Geometry: final body of the model. Coordinates: model frame, mm. A direction names the side the tool comes from. Give positions to 0.01 mm unless a question says otherwise; leave off trailing zeros. Loops run counter-clockwise (first coordinate to the right, second up) from the corner with the lowest first, then second, coordinate; pieces in that order, holes last. Notation, with made-up numbers: (19.25, 26) - (42.25, 26) arc R33 ccw to (42.25, 56) - close; hole circle Ø8 at (-2, -22.75). An arc over 180 degrees is marked (long way). Answer in a Markdown table with one row per item.
from build123d import *

# Parameters (mm, degrees)
F0_R     = 3.81
F1_DEPTH = 5.588
F2_DEPTH = 3.81
F3_R     = 1.5875
F4_DEPTH = 76.2
F5_SIZE  = 0.254
F6_SIZE  = 0.254


with BuildPart() as f1:
    # F0 (on Front) → F1 (new body)
    with BuildSketch(Plane.XZ):
        Circle(F0_R)
        Polygon((0, 2.54), (2.199705, 1.27), (2.199705, -1.27), (0, -2.54), (-2.199705, -1.27), (-2.199705, 1.27), align=None, mode=Mode.SUBTRACT)
    extrude(amount=F1_DEPTH)

    # F0 (on Front) → F2 (join)
    with BuildSketch(Plane.XZ):
        Polygon((2.199705, -1.27), (2.199705, 1.27), (0, 2.54), (-2.199705, 1.27), (-2.199705, -1.27), (0, -2.54), align=None)
    extrude(amount=F2_DEPTH)

    # F3 (on face) → F4 (join)
    with BuildSketch(Plane(origin=(0, 0, 0), x_dir=(-1, 0, 0), z_dir=(0, 1, 0))):
        Circle(F3_R)
    extrude(amount=F4_DEPTH)

    # F5
    f5_edges = [f1.edges().sort_by_distance(p)[0] for p in [
        (-3.81, -5.588, 0),
        (-3.81, 0, 0),
    ]]
    chamfer(f5_edges, length=F5_SIZE)

    # F6
    f6_edges = [f1.edges().sort_by_distance(p)[0] for p in [
        (1.5875, 76.2, 0),
    ]]
    chamfer(f6_edges, length=F6_SIZE)


solid = f1.part
Q1. Cut plane A-A (z = 0). Output: boundary loops of the cut face in (x, y), and give its area (4 significant figures).
Check values:
| item | result |
|---|---|
| outline | (-3.81, -5.33) - (-3.56, -5.59) - (-2.2, -5.59) - (-2.2, -3.81) - (2.2, -3.81) - (2.2, -5.59) - (3.56, -5.59) - (3.81, -5.33) - (3.81, -0.25) - (3.56, 0) - (1.59, 0) - (1.59, 75.95) - (1.33, 76.2) - (-1.33, 76.2) - (-1.59, 75.95) - (-1.59, 0) - (-3.56, 0) - (-3.81, -0.25) - close |
| area | 276.5 mm² |
Q2. Draft query along X for faces 4 (the cylindrical face through (0.34, 37.44, -1.55)), 5 (the flat face through (1.115, -4.687, -1.896)), 6 (the flat face through (0.74, -5.588, -2.32)). Return one class per face: pulls with the +X half, pulls with the -X half, needs draft (parallel to the pull), parting line crosses it, or undercut.
Check values:
| item | result |
|---|---|
| face 4 | parting line crosses it |
| face 5 | undercut |
| face 6 | needs draft |
Q3. First-contact query: pin 1 (3 mm diameter, centred on y = 61, z = -0.5, fed in from +X); pin 2 (1.5 mm diameter, centred on y = 6.5, z = -1, fed in from -X); pin 3 (0.9 mm diameter, centred on y = -4.5, z = -0.5, fed in from +X); pin 4 (4 mm diameter, centred on x = -3, y = 18.5, fed in from -Z). Flat tips, straight axial feed; report the tip coordinate or a pass-through.
Check values:
| item | result |
|---|---|
| pin 1 | x = 1.59 |
| pin 2 | x = -1.57 |
| pin 3 | x = 3.81 |
| pin 4 | z = -1.23 |
Q4. Reachability of faces 1 (the cylindrical face through (-0.83, -2.76, -3.72)), 2 (the flat face through (2, 0, -1)), 3 (the flat face through (2.2, -5, 0)) from +Z, -Z, +X, -X, +Y, -Y: full face, straight path, thin tool, end or side. Return the list, or none.
Check values:
| item | result |
|---|---|
| face 1 | +Y, -Y |
| face 2 | +Y |
| face 3 | -Y |
Q5. Material intervals for line 1 along Y through (x, z) = (0, 3); line 2 along Y through (x, z) = (-1.5, 1.5); line 3 along Z through (x, y) = (0, 24.5), sorted ascending.
Check values:
| item | result |
|---|---|
| line 1 | -5.59 to 0 |
| line 2 | -3.81 to 0 |
| line 3 | -1.59 to 1.59 |
Q6. Cut plane B-B (y = 70). Output: boundary loops of the cut face in (x, z) (1 decimal).
Check values:
| item | result |
|---|---|
| outline | circle Ø3.2 at (0, 0) |
